Geometry: final body of the model. Coordinates: model frame, mm. A direction names the side the tool comes from. Give positions to 0.01 mm unless a question says otherwise; leave off trailing zeros. Answer in a Markdown table with one row per item. Add a question column.
Q1. Line query: line 1 along X through (y, z) = (-9.5, 0.6); line 2 along X through (y, z) = (-10, 0.1); line 3 along X through (y, z) = (-16, 0.95). Output: solid intervals per line, ascending. Write a range as from..to.
Q2. Pull-direction query (X, two-part tool) for faces 3 (the face through (-1.5, -7.368, 0.5)), 4 (the face through (20.61, -10.59, 0.49)), 5 (the face through (16, -9.288, 0.5)); classes: +X half, -X half, draft (parallel to the pull), parting line (faces both ways), or undercut.
Q3. Set-up query: faces 1 (the face through (11.48, -10.76, 0.49)), 2 (the face through (16, -12, 1)). Return all of +Z, -Z, +X, -X, +Y, -Y with unobstructed straight access to the full face (end or side cutting, diameter ignored); none if empty.
from build123d import *

# Parameters (mm, degrees)
F2_DEPTH = 1
F3_T     = -1
F4_R     = 3.349925
F5_DEPTH = 25.4


with BuildPart() as f2:
    # F1 (on Top) → F2 (new body)
    with BuildSketch(Plane.XY):
        with BuildLine():
            Line((13.80021, -11.290746), (9.102559, -10.212597))
            add(Edge.make_bspline(
                [(9.102559, -10.212597), (8.142358, -10.075296), (7.32683, -8.968351), (6.992009, -7.368016)],
                knots=[0, 0, 0, 0, 3.542042, 3.542042, 3.542042, 3.542042], degree=3))
            Line((6.992009, -7.368016), (-10.196833, -7.368016))
            add(Edge.make_bspline(
                [(-10.196833, -7.368016), (-1.683224, -8.74827), (-0.829401, -13.403604), (-1.790936, -16.902696)],
                knots=[0, 0, 0, 0, 12.710989, 12.710989, 12.710989, 12.710989], degree=3))
            add(Edge.make_bspline(
                [(-1.790936, -16.902696), (5.33876, -16.336972), (13.023932, -16.339568), (15.948245, -24.916124)],
                knots=[0, 0, 0, 0, 19.465189, 19.465189, 19.465189, 19.465189], degree=3))
            add(Edge.make_bspline(
                [(15.948245, -24.916124), (19.640299, -16.68267), (25.902187, -16.389608), (33.941839, -17.028365)],
                knots=[0, 0, 0, 0, 19.64653, 19.64653, 19.64653, 19.64653], degree=3))
            add(Edge.make_bspline(
                [(33.941839, -17.028365), (30.768488, -9.431371), (40.071145, -8.176144), (42.985801, -7.154439)],
                knots=[0, 0, 0, 0, 13.389834, 13.389834, 13.389834, 13.389834], degree=3))
            Line((42.985801, -7.154439), (24.282036, -7.154439))
            add(Edge.make_bspline(
                [(24.282036, -7.154439), (24.807367, -8.005574), (24.392679, -9.044486), (23.041492, -10.058575)],
                knots=[0, 0, 0, 0, 3.157999, 3.157999, 3.157999, 3.157999], degree=3))
            Line((23.041492, -10.058575), (18.112808, -11.136725))
            add(Edge.make_bspline(
                [(18.112808, -11.136725), (16.990187, -10.975688), (17.650745, -9.288468), (17.419713, -8.36434)],
                knots=[0, 0, 0, 0, 2.857708, 2.857708, 2.857708, 2.857708], degree=3))
            Line((17.419713, -8.36434), (16.649606, -9.288468))
            Line((16.649606, -9.288468), (15.417434, -9.288468))
            Line((15.417434, -9.288468), (14.647327, -8.28733))
            add(Edge.make_bspline(
                [(14.647327, -8.28733), (14.364955, -9.288469), (14.845224, -10.811385), (13.80021, -11.290746)],
                knots=[0, 0, 0, 0, 3.120595, 3.120595, 3.120595, 3.120595], degree=3))
        make_face()
    extrude(amount=F2_DEPTH)

    # F3
    f3_openings = [f2.faces().sort_by_distance(p)[0] for p in [
        (16.284264, -13.143968, 1),
    ]]
    offset(amount=F3_T, openings=f3_openings)

    # F4 (on face) → F5 (cut)
    with BuildSketch(Plane.XY.offset(1)):
        with Locations((15.764091, -15.87615)):
            Circle(F4_R)
    extrude(amount=-F5_DEPTH, mode=Mode.SUBTRACT)


solid = f2.part
Completed:
| question | item | result |
|---|---|---|
| 1 | line 1 | x = -4.26..7.94, 14.53..17.45, 23.69..36.39 |
| 1 | line 2 | x = -3.62..8.52, 14.51..17.43, 23.12..35.61 |
| 1 | line 3 | x = -1.59..12.42, 19.11..33.58 |
| 2 | face 3 | draft |
| 2 | face 4 | undercut |
| 2 | face 5 | undercut |
| 3 | face 1 | +Z, -Z, +Y |
| 3 | face 2 | +Z, +X, -X, +Y, -Y |
